from build123d import *

# Parameters (mm, degrees)
F1_DEPTH = 5
F2_R     = 0.3


with BuildPart() as f1:
    # F0 (on Top) → F1 (new body, symmetric)
    with BuildSketch(Plane.XY):
        with BuildLine():
            ThreePointArc((2, 1.0307764064), (0, -2.25), (-2, 1.0307764064))
            add(Edge.make_bspline(
                [(-2, 1.0307764064), (-1.7928318797, 1.4327416027), (-1.4752005994, 2.7539357485), (-1.94238935, 3.6588384503), (-2.4898940219, 4.2405549061)],
                knots=[0, 0, 0, 0, 0.4856533037, 1, 1, 1, 1], degree=3))
            ThreePointArc((-2.4898940219, 4.2405549061), (-2.9846417573, 4.255544178), (-2.9996310293, 3.7607964426))
            add(Edge.make_bspline(
                [(-2.6222222222, 1.3514623995), (-2.5879840781, 1.4178941569), (-2.5120919735, 1.5965615902), (-2.4185643331, 1.9365442889), (-2.3646202091, 2.2979855215), (-2.3625995138, 2.6240888033), (-2.4081716924, 2.8742683693), (-2.5044815542, 3.1179920879), (-2.6847308977, 3.4036360851), (-2.8805852991, 3.6343119324), (-2.9996310293, 3.7607964426)],
                knots=[0, 0, 0, 0, 0.125, 0.25, 0.375, 0.5, 0.625, 0.75, 0.875, 1, 1, 1, 1], degree=3))
            ThreePointArc((-2.6222222222, 1.3514623995), (-2.6973313466, -1.1945307057), (-0.7615773106, -2.85))
            Line((-0.7615773106, -2.85), (0.7615773106, -2.85))
            ThreePointArc((0.7615773106, -2.85), (2.6973313466, -1.1945307057), (2.6222222222, 1.3514623995))
            add(Edge.make_bspline(
                [(2.6222222222, 1.3514623995), (2.5879840781, 1.4178941569), (2.5120919735, 1.5965615902), (2.4185643331, 1.9365442889), (2.3646202091, 2.2979855215), (2.3625995138, 2.6240888033), (2.4081716924, 2.8742683693), (2.5044815542, 3.1179920879), (2.6847308977, 3.4036360851), (2.8805852991, 3.6343119324), (2.9996310293, 3.7607964426)],
                knots=[0, 0, 0, 0, 0.125, 0.25, 0.375, 0.5, 0.625, 0.75, 0.875, 1, 1, 1, 1], degree=3))
            ThreePointArc((2.9996310293, 3.7607964426), (2.9846417573, 4.255544178), (2.4898940219, 4.2405549061))
            add(Edge.make_bspline(
                [(2, 1.0307764064), (1.7928318797, 1.4327416027), (1.4752005994, 2.7539357485), (1.94238935, 3.6588384503), (2.4898940219, 4.2405549061)],
                knots=[0, 0, 0, 0, 0.4856533037, 1, 1, 1, 1], degree=3))
        make_face()
        with BuildLine():
            ThreePointArc((0.7615773106, -2.85), (0, -2.95), (-0.7615773106, -2.85))
            Line((-0.7615773106, -2.85), (-6, -2.85))
            Line((-6, -2.85), (-6, -3.85))
            Line((-6, -3.85), (6, -3.85))
            Line((6, -3.85), (6, -2.85))
            Line((6, -2.85), (0.7615773106, -2.85))
        make_face()
        with BuildLine():
            Line((0.7615773106, -2.85), (-0.7615773106, -2.85))
            ThreePointArc((-0.7615773106, -2.85), (0, -2.95), (0.7615773106, -2.85))
        make_face()
    extrude(amount=F1_DEPTH, both=True)

    # F2
    f2_edges = [f1.edges().sort_by_distance(p)[0] for p in [
        (-6, -2.85, 0),
        (-6, -3.85, 0),
        (6, -2.85, 0),
        (6, -3.85, 0),
        (0.761577, -2.85, 0),
        (-0.761577, -2.85, 0),
    ]]
    fillet(f2_edges, radius=F2_R)


solid = f1.part
Can you work these out from the model? Positions are in its coordinate system, mm. A direction names the side the tool comes from. Coordinates: 2 decimals unless noted, no trailing zeros. Order: outer loops, then holes, each group sorted by start corner. A loop starts at its lowest first (then second) coordinate and runs counter-clockwise, first axis right, second up. Notation, with made-up numbers: (24, 56.25) -> (42, 56.25) arc R29 cw to (42, 92.25) -> close; hole circle Ø1 at (-12, 0.5). An arc over 180 degrees is marked (long way). Use one line per item in the form item = value.
Q1. I need wall thicknesses on L1, parallel to X at y = 0, z = -2; L2, parallel to Y at x = -3.5, z = 3.5; L3, parallel to X at y = -1.75, z = -3.25. Which ranges of each line are inside material? Lowest first, please.
From the geometry:
L1 = -2.95 to -2.25, 2.25 to 2.95
L2 = -3.85 to -2.85
L3 = -2.37 to -1.41, 1.41 to 2.37
Q2. Imagine slicing it at B-B, the plane x = 3.75. List the corners of the cut face in (y, z) for me, then the cut area to 4 significant figures.
From the geometry:
outline = (-3.85, -5) -> (-2.85, -5) -> (-2.85, 5) -> (-3.85, 5) -> close
area = 10.00 mm²
Q3. We'd pull the mould along Y, two halves only. Please class faces 1 (the face through (0, -3.85, 0)), 2 (the face through (0, -2.5, 5)), 3 (the face through (2.877, -0.652, 0.07)): released by +Y, released by -Y, zero draft, split by the parting line, or undercut.
From the geometry:
face_1 = released by -Y
face_2 = zero draft
face_3 = undercut
Q4. Will these pins go through, and if not, where does the flat tip stop? P1, Ø3.5, axis at x = 0, y = 0, coming from the +Z side; P2, Ø4, axis at x = -3.5, y = 1.5, coming from the -Z side.
From the geometry:
P1 = through
P2 = -5
Q5. Which directions (+Z, -Z, +X, -X, +Y, -Y) give clear straight access to the entire face, cutting with the end or side of a thin tool? Please do faces 4 (the face through (-4, -2.85, 0)), 5 (the face through (0, -2.5, -5)), 6 (the face through (4, -2.85, 0)).
From the geometry:
face_4 = +Z, -Z, -X
face_5 = -Z, +X, -X, +Y, -Y
face_6 = +Z, -Z, +X
Q6. Imagine slicing it at A-A, the plane y = 0. List the corners of the cut face in (x, z) for me.
From the geometry:
outline = (-2.95, -5) -> (-2.25, -5) -> (-2.25, 5) -> (-2.95, 5) -> close; (2.25, -5) -> (2.95, -5) -> (2.95, 5) -> (2.25, 5) -> close
Q7. Imagine slicing it at C-C, the plane x = 0. List the corners of the cut face in (y, z) for me.
From the geometry:
outline = (-3.85, -5) -> (-2.25, -5) -> (-2.25, 5) -> (-3.85, 5) -> close
